Verification items for the finished model (mm, model axes). A direction names the side the tool comes from. Coordinates: 2 decimals unless noted, no trailing zeros. Order: outer loops, then holes, each group sorted by start corner. A loop starts at its lowest first (then second) coordinate and runs counter-clockwise, first axis right, second up. Notation, with made-up numbers: M 84,37 L 99,37 A30 ccw 99,74 Z; hole C 46,78.25 d9. An arc over 180 degrees is marked long. Answer as a JSON object with one key per item and string values. Group by question number.
(1) Cross-section at D-D (x = -8). Enter the section's corners in (y, z) (3 decimals), plus the area to 3 significant figures.
(2) Cross-section at B-B (y = -12.7). Enter the section's corners in (x, z) (3 decimals).
(3) Cross-section at C-C (x = -23.5). Enter the section's corners in (y, z) (3 decimals).
(4) Cross-section at A-A (z = 3.75). Enter the section's corners in (x, y), plus the area to 3 significant figures.
(5) Mould release check, pull along X, two halves, no side actions. Record for faces 4 (the face through (-13, 0, 4)), 5 (the face through (-25.337, -18.054, 4.383)), 6 (the face through (-12, -13, 8.89)), 7 (the face through (10.868, -2.173, 5.053)): released by +X, released by -X, zero draft, split by the parting line, or undercut.
(6) Access from +Z, -Z, +X, -X, +Y, -Y to the whole of each face (thin tool, end or side, straight path). Record for faces 1 (the face through (-5.6, -12.5, 0)), 2 (the face through (10.986, -23.109, 5.053)), 3 (the face through (-29, -13, 8.89)).
(7) Gauge pin test, flat ends, axial feed: pin 1 Ø5 at (y, z) = (-18, 7) entering from +X; pin 2 Ø5 at (y, z) = (-21, 6.5) entering from -X; pin 3 Ø10 at (x, y) = (-27.5, -12) entering from -Z; pin 4 Ø2.5 at (x, y) = (16.33, -6.35) entering from -Z. Record the tip position at first contact, or that the pin passes through.
(8) Material ranges on line 1 (X direction, y = -12.7, z = 5.5); line 2 (X direction, y = -16.25, z = 7.5); line 3 (Z direction, x = 2.5, y = -10.25) (3 decimals), recorded low to high.
from build123d import *

# Parameters (mm, degrees)
F1_DEPTH     = 25.4
F3_R         = 1.651
F4_DEPTH     = 3.176
F5_R         = 6.35
F6_DEPTH     = 8.89
F7_R         = 5.08
F8_R         = 2.54
F9_T1_DEPTH  = 6.35
F9_T4_ANGLE  = 90
F9_T6_ANGLE  = 90
F9_T8_ANGLE  = 90
F9_T10_ANGLE = 90


# Not quite as in the source:
# - a fillet or chamfer that OpenCascade refuses, or shapes differently, is made with other operations: its cross-section is extruded or revolved along the edge and cut away or added
# - a feature names something its author has since deleted; it is built from what else it names


with BuildPart() as f1:
    # F0 (on Front) → F1 (new body)
    with BuildSketch(Plane.XZ):
        Polygon((-43.9910670578, 3.175), (-43.9910670578, 0), (19.5089329422, 0), (19.5089329422, 3.175), (13.1589329422, 3.175), (13.1589329422, 9.525), (-37.6410670578, 9.525), (-37.6410670578, 3.175), align=None)
    extrude(amount=F1_DEPTH)

    # F3 (on face) → F4 (cut, through all)
    with BuildSketch(Plane.XY.offset(3.175)):
        with Locations((-40.8160670578, -19.05)):
            Circle(F3_R)
        with Locations((-40.8160670578, -6.35)):
            Circle(F3_R)
        with Locations((16.3339329422, -6.35)):
            Circle(F3_R)
        with Locations((16.3339329422, -19.05)):
            Circle(F3_R)
    extrude(amount=-F4_DEPTH, mode=Mode.SUBTRACT)

    # F5 (on face) → F6 (cut)
    with BuildSketch(Plane(origin=(0, 0, 0), x_dir=(1, 0, 0), z_dir=(0, 0, -1))):
        with Locations((-28.7510670578, 12.7)):
            Circle(F5_R)
        with Locations((4.2689329422, 12.7)):
            Circle(F5_R)
        with Locations((-12.2410670578, 12.7)):
            Circle(F5_R)
    extrude(amount=-F6_DEPTH, mode=Mode.SUBTRACT)

    # F7
    f7_edges = [f1.edges().sort_by_distance(p)[0] for p in [
        (19.508933, -25.4, 1.5875),
        (19.508933, 0, 1.5875),
        (-43.991067, -25.4, 1.5875),
        (-43.991067, 0, 1.5875),
    ]]
    fillet(f7_edges, radius=F7_R)

    # F8
    f8_edges = [f1.edges().sort_by_distance(p)[0] for p in [
        (-12.241067, -25.4, 9.525),
        (-37.641067, -12.7, 9.525),
        (-12.241067, 0, 9.525),
        (13.158933, -12.7, 9.525),
    ]]
    fillet(f8_edges, radius=F8_R)

    # F9: fillet of radius 7.62 on 4 edges, made by hand

    # F9_s2 → F9_t1 (cut)
    with BuildSketch(Plane.XY.offset(3.175)):
        with BuildLine():
            ThreePointArc((-37.6410670578, -17.78), (-35.4092207305, -23.1681536726), (-30.0210670578, -25.4))
            Line((-30.0210670578, -25.4), (-37.6410670578, -25.4))
            Line((-37.6410670578, -25.4), (-37.6410670578, -17.78))
        make_face()
        with BuildLine():
            ThreePointArc((13.1589329422, -17.78), (10.9270866148, -23.1681536726), (5.5389329422, -25.4))
            Line((5.5389329422, -25.4), (13.1589329422, -25.4))
            Line((13.1589329422, -25.4), (13.1589329422, -17.78))
        make_face()
        with BuildLine():
            ThreePointArc((-30.0210670578, 0), (-35.4092207305, -2.2318463274), (-37.6410670578, -7.62))
            Line((-37.6410670578, -7.62), (-37.6410670578, 0))
            Line((-37.6410670578, 0), (-30.0210670578, 0))
        make_face()
        with BuildLine():
            ThreePointArc((5.5389329422, 0), (10.9270866148, -2.2318463274), (13.1589329422, -7.62))
            Line((13.1589329422, -7.62), (13.1589329422, 0))
            Line((13.1589329422, 0), (5.5389329422, 0))
        make_face()
    extrude(amount=F9_T1_DEPTH, mode=Mode.SUBTRACT)

    # F9_s3 → F9_t4 (revolve, cut)
    with BuildSketch(Plane.XZ.offset(7.62)):
        with BuildLine():
            ThreePointArc((10.6189329422, 9.525), (12.4149841664, 8.7810512242), (13.1589329422, 6.985))
            Line((13.1589329422, 6.985), (13.1589329422, 9.525))
            Line((13.1589329422, 9.525), (10.6189329422, 9.525))
        make_face()
    revolve(axis=Axis((5.5389329422, -7.62, 9.525), (0, 0, 1)), revolution_arc=F9_T4_ANGLE, mode=Mode.SUBTRACT)

    # F9_s5 → F9_t6 (revolve, cut)
    with BuildSketch(Plane.YZ.offset(-30.0210670578)):
        with BuildLine():
            ThreePointArc((-2.54, 9.525), (-0.7439487758, 8.7810512242), (0, 6.985))
            Line((0, 6.985), (0, 9.525))
            Line((0, 9.525), (-2.54, 9.525))
        make_face()
    revolve(axis=Axis((-30.0210670578, -7.62, 9.525), (0, 0, 1)), revolution_arc=F9_T6_ANGLE, mode=Mode.SUBTRACT)

    # F9_s7 → F9_t8 (revolve, cut)
    with BuildSketch(Plane.YZ.offset(5.5389329422)):
        with BuildLine():
            ThreePointArc((-22.86, 9.525), (-24.6560512242, 8.7810512242), (-25.4, 6.985))
            Line((-25.4, 6.985), (-25.4, 9.525))
            Line((-25.4, 9.525), (-22.86, 9.525))
        make_face()
    revolve(axis=Axis((5.5389329422, -17.78, 9.525), (0, 0, 1)), revolution_arc=F9_T8_ANGLE, mode=Mode.SUBTRACT)

    # F9_s9 → F9_t10 (revolve, cut)
    with BuildSketch(Plane.XZ.offset(17.78)):
        with BuildLine():
            ThreePointArc((-35.1010670578, 9.525), (-36.8971182821, 8.7810512242), (-37.6410670578, 6.985))
            Line((-37.6410670578, 6.985), (-37.6410670578, 9.525))
            Line((-37.6410670578, 9.525), (-35.1010670578, 9.525))
        make_face()
    revolve(axis=Axis((-30.0210670578, -17.78, 9.525), (0, 0, 1)), revolution_arc=F9_T10_ANGLE, mode=Mode.SUBTRACT)


solid = f1.part
Taken from the geometry:
{
 "1": {"outline": "M -25.4,0 L -17.426,0 L -17.426,8.89 L -7.974,8.89 L -7.974,0 L 0,0 L 0,6.985 A2.54 ccw -2.54,9.525 L -22.86,9.525 A2.54 ccw -25.4,6.985 Z", "area": "155 mm²"},
 "2": {"outline": "M -43.991,0 L -35.101,0 L -35.101,8.89 L -22.401,8.89 L -22.401,0 L -18.591,0 L -18.591,8.89 L -5.891,8.89 L -5.891,0 L -2.081,0 L -2.081,8.89 L 10.619,8.89 L 10.619,0 L 19.509,0 L 19.509,3.175 L 13.159,3.175 L 13.159,6.985 A2.54 ccw 10.619,9.525 L -35.101,9.525 A2.54 ccw -37.641,6.985 L -37.641,3.175 L -43.991,3.175 Z"},
 "3": {"outline": "M -25.4,0 L -16.271,0 L -16.271,8.89 L -9.129,8.89 L -9.129,0 L 0,0 L 0,6.985 A2.54 ccw -2.54,9.525 L -22.86,9.525 A2.54 ccw -25.4,6.985 Z"},
 "4": {"outline": "M -37.64,-17.78 A7.62 ccw -30.02,-25.4 L 5.54,-25.4 A7.62 ccw 13.16,-17.78 L 13.16,-7.62 A7.62 ccw 5.54,0 L -30.02,0 A7.62 ccw -37.64,-7.62 Z; hole C -28.75,-12.7 d12.7; hole C -12.24,-12.7 d12.7; hole C 4.27,-12.7 d12.7", "area": "860 mm²"},
 "5": {"face 4": "zero draft", "face 5": "undercut", "face 6": "undercut", "face 7": "released by +X"},
 "6": {"face 1": "-Z, +X, -X, +Y, -Y", "face 2": "+Z, +X, -Y", "face 3": "-Z"},
 "7": {"pin 1": "stops at x = 13.16", "pin 2": "stops at x = -37.61", "pin 3": "stops at z = 0", "pin 4": "passes through"},
 "8": {"line 1": "x = -37.64 to -35.1, -22.4 to -18.59, -5.89 to -2.08, 10.62 to 13.16", "line 2": "x = -37.59 to -34.02, -23.49 to -17.51, -6.98 to -1, 9.53 to 13.11", "line 3": "z = 8.89 to 9.525"}
}
